from build123d import *

# Parameters (mm, degrees)
SKETCH1_W           = 42
SKETCH1_H           = 52
BOSS_EXTRUDE1_DEPTH = 3
SKETCH2_R           = 19
CUT_EXTRUDE1_DEPTH  = 7
SKETCH3_R           = 1.2
CUT_EXTRUDE2_DEPTH  = 8
SKETCH4_R           = 1.2
CUT_EXTRUDE3_DEPTH  = 8


with BuildPart() as part:
    # Sketch1 → Boss-Extrude1 (new body, symmetric)
    with BuildSketch(Plane(origin=(0, 0, 0), x_dir=(1, 0, 0), z_dir=(0, 1, 0))):
        Rectangle(SKETCH1_W, SKETCH1_H)
    extrude(amount=BOSS_EXTRUDE1_DEPTH, both=True)

    # Sketch2 → Cut-Extrude1 (cut, through all)
    with BuildSketch(Plane(origin=(0, 3, 0), x_dir=(1, 0, 0), z_dir=(0, 1, 0))):
        Circle(SKETCH2_R)
    extrude(amount=-CUT_EXTRUDE1_DEPTH, mode=Mode.SUBTRACT)

    # Sketch3 → Cut-Extrude2 (cut)
    with BuildSketch(Plane(origin=(0, 0, -26), x_dir=(-1, 0, 0), z_dir=(0, 0, -1))):
        with Locations((-15, 0)):
            Circle(SKETCH3_R)
        with Locations((15, 0)):
            Circle(SKETCH3_R)
    extrude(amount=-CUT_EXTRUDE2_DEPTH, mode=Mode.SUBTRACT)

    # Sketch4 → Cut-Extrude3 (cut)
    with BuildSketch(Plane.XY.offset(26)):
        with Locations((15, 0)):
            Circle(SKETCH4_R)
        with Locations((-15, 0)):
            Circle(SKETCH4_R)
    extrude(amount=-CUT_EXTRUDE3_DEPTH, mode=Mode.SUBTRACT)


solid = part.part
The listing builds one solid part. Answer for the finished solid, in the listing's coordinates (mm). A direction names the side the tool comes from. Coordinates: 2 decimals unless noted, no trailing zeros. Write each loop counter-clockwise with the first axis right and the second up, starting at its lowest first coordinate (ties: lowest second). Pieces come first, ordered by that corner, then holes. Notation, with made-up numbers: M -19,-27.75 L 4,-27.75 A21 ccw 4,-23.75 Z; hole C 28,16 d2. An arc over 180 degrees is marked long. Put each result on its own line as item: value. Start each with the question number.
1. Consider line 1 (X direction, y = 0.6, z = 21.5); line 2 (Z direction, x = -0.5, y = -1.3); line 3 (Y direction, x = 15, z = 21.5). Determine where each line is inside the solid, lowest interval first. Write a range as from..to.
2. A cutting plane is placed at A-A on x = 0. Write down the section's boundary in (y, z).
3. Flat-ended cylindrical pins translate along their axes: P1, Ø0.7, axis at x = -15.5, y = 0.5, coming from the -Z side; P2, Ø1.9, axis at x = -15, y = 0, coming from the +Z side. Find the tip coordinate at first contact, or state that the pin passes through.
4. A cutting plane is placed at B-B on y = 0. Write down the section's boundary in (x, z).
5. Which of the six approach directions +Z, -Z, +X, -X, +Y, -Y give full straight-line access (tool end or side, diameter ignored) to faces 4 (the flat face through (-15, 0, 18)), 5 (the flat face through (-21, 0, 0)), 6 (the flat face through (15, 0, -18))?
6. For a pull along Y with two mould halves and no side action, classify faces 1 (the flat face through (15, 0, 18)), 2 (the flat face through (0, 0, -26)), 3 (the flat face through (18.4, -3, -6.1)) as pulls with the +Y half, pulls with the -Y half, needs draft (parallel to the pull), parting line crosses it, or undercut.
7. A cutting plane is placed at D-D on z = 2. Write down the section's boundary in (x, y).
8. A cutting plane is placed at C-C on z = 23.5. Write down the section's boundary in (x, y), then the cut area to 3 significant figures.
Resolved:
1. line 1: x = -21..-16.04, -13.96..13.96, 16.04..21
1. line 2: z = -26..-18.99, 18.99..26
1. line 3: y = -3..-1.2, 1.2..3
2. outline: M -3,-26 L 3,-26 L 3,-19 L -3,-19 Z; M -3,19 L 3,19 L 3,26 L -3,26 Z
3. P1: stops at z = -18
3. P2: stops at z = 18
4. outline: M -21,-26 L -16.2,-26 L -16.2,-18 L -13.8,-18 L -13.8,-26 L 13.8,-26 L 13.8,-18 L 16.2,-18 L 16.2,-26 L 21,-26 L 21,26 L 16.2,26 L 16.2,18 L 13.8,18 L 13.8,26 L -13.8,26 L -13.8,18 L -16.2,18 L -16.2,26 L -21,26 Z; hole C 0,0 d38
5. face 4: +Z
5. face 5: +Z, -Z, -X, +Y, -Y
5. face 6: -Z
6. face 1: undercut
6. face 2: needs draft
6. face 3: pulls with the -Y half
7. outline: M -21,-3 L -18.89,-3 L -18.89,3 L -21,3 Z; M 18.89,-3 L 21,-3 L 21,3 L 18.89,3 Z
8. outline: M -21,-3 L 21,-3 L 21,3 L -21,3 Z; hole C -15,0 d2.4; hole C 15,0 d2.4
8. area: 243 mm2
